The model under review builds one solid part; all positions refer to its coordinate system, in mm. A direction names the side the tool comes from. Give positions to 0.01 mm unless a question says otherwise; leave off trailing zeros. Loops run counter-clockwise (first coordinate to the right, second up) from the corner with the lowest first, then second, coordinate; pieces in that order, holes last. Notation, with made-up numbers: M 3.25,21 L 27.25,21 A24 ccw 27.25,50 Z; hole C 81.5,40 d2. An arc over 180 degrees is marked long. Write item = value, one per line. Start each with the question number.
1. For pin 1 (2 mm diameter, centred on y = 2.5, z = 1.5, fed in from -X); pin 2 (1 mm diameter, centred on y = 3.5, z = -3, fed in from -X); pin 3 (2 mm diameter, centred on y = 4.5, z = -3, fed in from +X), all flat-tipped, find the tip position at first contact; note any pin that passes through.
2. We need section C-C on y = 7.25. Give the boundary of the cut face in (x, z) (3 decimals), then the cut area to 3 significant figures.
3. We need section D-D on y = 1.25. Give the boundary of the cut face in (x, z) (3 decimals), then the cut area to 3 significant figures.
4. For faces 4 (the face through (-2.74, 7.11, 2.51)), 5 (the face through (2, 8.8, 2)), list the 3-axis set-ups (+Z, -Z, +X, -X, +Y, -Y) from which the entire face can be reached by the end or side of a thin tool; tool diameter is ignored.
5. Wall thickness on line 1 along Z through (x, y) = (0, 3.25) (3 decimals); line 2 along Z through (x, y) = (0, 5.5) (3 decimals); line 3 along X through (y, z) = (1, -1.25): over which ranges is each line inside the solid? List them lowest first. Write a range as from..to.
6. We need section A-A on x = 0. Give the boundary of the cut face in (y, z) (3 decimals).
7. Draft analysis for pull direction Z (two halves, no side actions). For faces 1 (the face through (-0.542, 4.462, 1.726)), 2 (the face through (0.878, 2.465, 3.954)), 3 (the face through (0, 0, 2)), state which applies: pulls with the +Z half, pulls with the -Z half, needs draft (parallel to the pull), parting line crosses it, or undercut.
8. We need section B-B on z = 0. Give the boundary of the cut face in (x, y) (3 decimals), then the cut area to 3 significant figures.
Autodesk Inventor part; units mm, degrees
ref_plane "YZ Plane" through (0, 0, 0) normal (1, 0, 0) x (0, 1, 0)
ref_plane "XZ Plane" through (0, 0, 0) normal (0, 1, 0) x (-1, 0, 0)
ref_plane "XY Plane" through (0, 0, 0) normal (0, 0, 1) x (1, 0, 0)
sketch "Boceto1" plane through (0, 0, 0) normal (0, 1, 0) x (-1, 0, 0)
  circle A0 centre (0, 0) radius 4.05
  dimension "d0" = 8.1
extrude "Extrusión1" add sketch "Boceto1" along normal blind 5
sketch "Boceto2" plane through (0, 5, 0) normal (0, 1, 0) x (1, 0, 0)
  circle A0 centre (0, 0) radius 3.715
  dimension "d3" = 7.43
extrude "Extrusión2" add sketch "Boceto2" along normal blind 3.8
fillet "Empalme2" radius 0.5 1 edges at (-3.715, 5, 0)
sketch "Boceto14" plane through (0, 8.8, 0) normal (0, 1, 0) x (1, 0, 0)
  circle A0 centre (0, 0) radius 3.715
  line L0 (0, 3.715) -> (0, 3.215)
  line L1 (0, 3.215) -> (0, 0.715)
  circle A1 centre (0, 0.715) radius 2.5
  dimension "d72" = 0.5
  dimension "d73" = 2.5
extrude "Extrusión7" cut sketch "Boceto14" against normal through all contours A1
equation "\"d23\" = 55deg"
equation "\"Boceto5_Pitch\" = 0.8"
equation "\"d45\" = 55deg"
equation "\"Boceto8_Pitch\" = 0.8"
properties part number "interior"
Final values:
q1.pin_1 = -4.02
q1.pin_2 = -3.19
q1.pin_3 = 3.52
q2.outline = C 0,0 d7.43; hole C 0,-0.715 d5
q2.area = 23.7 mm²
q3.outline = C 0,0 d8.1; hole C 0,-0.715 d5
q3.area = 31.9 mm²
q4.face_4 = +Y
q4.face_5 = +Z, -Z, +X, -X, +Y
q5.line_1 = -4.05..-3.215, 1.785..4.05
q5.line_2 = -3.715..-3.215, 1.785..3.715
q5.line_3 = -3.85..-2.44, 2.44..3.85
q6.outline = M 0,-4.05 L 5,-4.05 A0.5 cw 5.472,-3.715 L 8.8,-3.715 L 8.8,-3.215 L 0,-3.215 Z; M 0,1.785 L 8.8,1.785 L 8.8,3.715 L 5.472,3.715 A0.5 cw 5,4.05 L 0,4.05 Z
q7.face_1 = undercut
q7.face_2 = parting line crosses it
q7.face_3 = needs draft
q8.outline = M -4.05,0 L -2.396,0 L -2.396,8.8 L -3.715,8.8 L -3.715,5.472 A0.5 cw -4.05,5 Z; M 2.396,0 L 4.05,0 L 4.05,5 A0.5 cw 3.715,5.472 L 3.715,8.8 L 2.396,8.8 Z
q8.area = 26.7 mm²
